Here's how the part is built. I have some questions about the finished solid (model axes, mm). A direction names the side the tool comes from. Give positions to 0.01 mm unless a question says otherwise; leave off trailing zeros. Write each loop counter-clockwise with the first axis right and the second up, starting at its lowest first coordinate (ties: lowest second). Pieces come first, ordered by that corner, then holes. Notation, with made-up numbers: (15.5, 23.5) -> (57.5, 23.5) arc R22 ccw to (57.5, 57.5) -> close; hole circle Ø4 at (-23, -29). An arc over 180 degrees is marked (long way). Use one line per item in the form item = value.
```python
from build123d import *

# Parameters (mm, degrees)
SKETCH_1_R          = 6
EXTRUDE_1_DEPTH     = 16
EXTRUDE_START       = 4
EXTRUDE_6_DEPTH     = 8
SKETCH_9_R          = 5
EXTRUDE_7_DEPTH     = 7
EXTRUDE_START_2     = -23
SKETCH_9_2_R        = 5
EXTRUDE_8_DEPTH     = 7
SKETCH_11_R         = 2
CUT_EXTRUDE_1_DEPTH = 33.511536414


with BuildPart() as part:
    # 草图1 → 凸台-拉伸1 (new body)
    with BuildSketch(Plane.XY):
        Circle(SKETCH_1_R)
    extrude(amount=EXTRUDE_1_DEPTH)

    # 草图8 → 凸台-拉伸6 (add)
    with BuildSketch(Plane.XY.offset(EXTRUDE_START)):
        with BuildLine():
            Line((10.5, 0.866025404), (3, 5.196152423))
            ThreePointArc((3, 5.196152423), (6, 0), (3, -5.196152423))
            Line((3, -5.196152423), (10.5, -0.866025404))
            ThreePointArc((10.5, -0.866025404), (11, 0), (10.5, 0.866025404))
        make_face()
        with BuildLine():
            Line((-10.5, -0.866025404), (-3, -5.196152423))
            ThreePointArc((-3, -5.196152423), (-6, 0), (-3, 5.196152423))
            Line((-3, 5.196152423), (-10.5, 0.866025404))
            ThreePointArc((-10.5, 0.866025404), (-11, 0), (-10.5, -0.866025404))
        make_face()
    extrude(amount=EXTRUDE_6_DEPTH)

    # 草图9 → 凸台-拉伸7 (add)
    with BuildSketch(Plane.XY.offset(16)):
        Circle(SKETCH_9_R)
    extrude(amount=EXTRUDE_7_DEPTH)

    # 草图9<2> → 凸台-拉伸8 (add)
    with BuildSketch(Plane.XY.offset(16).offset(EXTRUDE_START_2)):
        Circle(SKETCH_9_2_R)
    extrude(amount=EXTRUDE_8_DEPTH)

    # 草图11 → 切除-拉伸1 (cut, through all)
    with BuildSketch(Plane.XY.offset(23)):
        Circle(SKETCH_11_R)
    extrude(amount=-CUT_EXTRUDE_1_DEPTH, mode=Mode.SUBTRACT)


solid = part.part
```
Q1. Which directions (+Z, -Z, +X, -X, +Y, -Y) give clear straight access to the entire face, cutting with the end or side of a thin tool? Please do faces 1 (the face through (-4, 4, 16)), 2 (the face through (2.769, -5.323, 7.888)), 3 (the face through (-4, 4, 0)).
Result set:
face_1 = +Z
face_2 = none
face_3 = -Z
Q2. I want a section at A-A, the plane x = 0. Write out the boundary of the cut face in (y, z), and give its area (3 significant figures).
Result set:
outline = (-6, 0) -> (-5, 0) -> (-5, -7) -> (-2, -7) -> (-2, 23) -> (-5, 23) -> (-5, 16) -> (-6, 16) -> close; (2, -7) -> (5, -7) -> (5, 0) -> (6, 0) -> (6, 16) -> (5, 16) -> (5, 23) -> (2, 23) -> close
area = 212 mm2
Q3. If I drill on line 1 along Y through (x, z) = (0, 14.75); line 2 along X through (y, z) = (4, -4); line 3 along Y through (x, z) = (1.25, 3), over which ranges is the centre line in solid material (lowest first)? Write a range as from..to.
Result set:
line_1 = -6..-2, 2..6
line_2 = -3..3
line_3 = -5.87..-1.56, 1.56..5.87
Q4. I want a section at B-B, the plane y = 0. Write out the boundary of the cut face in (x, z).
Result set:
outline = (-11, 4) -> (-6, 4) -> (-6, 0) -> (-5, 0) -> (-5, -7) -> (-2, -7) -> (-2, 23) -> (-5, 23) -> (-5, 16) -> (-6, 16) -> (-6, 12) -> (-11, 12) -> close; (2, -7) -> (5, -7) -> (5, 0) -> (6, 0) -> (6, 4) -> (11, 4) -> (11, 12) -> (6, 12) -> (6, 16) -> (5, 16) -> (5, 23) -> (2, 23) -> close
Q5. I want a section at D-D, the plane y = -2.75. Write out the boundary of the cut face in (x, z).
Result set:
outline = (-7.24, 4) -> (-5.33, 4) -> (-5.33, 0) -> (-4.18, 0) -> (-4.18, -7) -> (4.18, -7) -> (4.18, 0) -> (5.33, 0) -> (5.33, 4) -> (7.24, 4) -> (7.24, 12) -> (5.33, 12) -> (5.33, 16) -> (4.18, 16) -> (4.18, 23) -> (-4.18, 23) -> (-4.18, 16) -> (-5.33, 16) -> (-5.33, 12) -> (-7.24, 12) -> close
Q6. If we mould it in two halves opening along Y, with no side actions, what happens to faces 4 (the face through (7, 0, 4)), 5 (the face through (0, -2, 8)), 6 (the face through (6.7, -3.06, 7.94))? For each: +Y half, -Y half, draft (parallel to the pull), parting line (faces both ways), or undercut.
Result set:
face_4 = draft
face_5 = undercut
face_6 = -Y half
Q7. Will these pins go through, and if not, where does the flat tip stop? pin 1 Ø1 at (x, y) = (-5.5, -3) entering from +Z; pin 2 Ø6 at (x, z) = (4.5, 5) entering from +Y; pin 3 Ø2.5 at (x, y) = (0, 0) entering from -Z; pin 4 Ø5 at (x, z) = (-7.5, 13.5) entering from +Y.
Result set:
pin_1 = 16
pin_2 = 5.81
pin_3 = through
pin_4 = 3.75
Q8. I want a section at C-C, the plane z = 7. Write out the boundary of the cut face in (x, y).
Result set:
outline = (-10.5, -0.87) -> (-3, -5.2) arc R6 ccw to (3, -5.2) -> (10.5, -0.87) arc R1 ccw to (10.5, 0.87) -> (3, 5.2) arc R6 ccw to (-3, 5.2) -> (-10.5, 0.87) arc R1 ccw to start; hole circle Ø4 at (0, 0)
